from build123d import *

# Parameters (mm, degrees)
REVOLVE_1_ANGLE             = 75
HOLE_WIZARD_M31_D           = 3.4
HOLE_WIZARD_M31_CBORE_D     = 6.05
HOLE_WIZARD_M31_CBORE_DEPTH = 3
FILLET_1_R                  = 2


with BuildPart() as part:
    # Эскиз1 → Повернуть1 (revolve)
    with BuildSketch(Plane.XY):
        Polygon((-52, 0), (-38.5, 0), (-38.5, 5.5), (-48, 5.5), (-48, 10), (-52, 10), align=None)
    revolve(axis=Axis((0, 0, 0), (0, -1, 0)), revolution_arc=REVOLVE_1_ANGLE)

    # Цековка для винта с заклепочной головкой M31 (through all)
    with Locations(Plane(origin=(0, 5.5, 0), x_dir=(1, 0, 0), z_dir=(0, 1, 0))):
        with Locations((-20.75, 35.940054257), (-40.085921791, 10.740990372)):
            CounterBoreHole(HOLE_WIZARD_M31_D / 2, HOLE_WIZARD_M31_CBORE_D / 2, HOLE_WIZARD_M31_CBORE_DEPTH)

    # Скругление1
    fillet_1_edges = [part.edges().sort_by_distance(p)[0] for p in [
        (-9.964533236, 2.75, -37.188144312),
        (-13.458590345, 5, -50.228142967),
        (-52, 5, 0),
        (-38.5, 2.75, 0),
    ]]
    fillet(fillet_1_edges, radius=FILLET_1_R)


solid = part.part
Part model, mm, in its own coordinate system. A direction names the side the tool comes from. Give positions to 0.01 mm unless a question says otherwise; leave off trailing zeros. Order: outer loops, then holes, each group sorted by start corner. A loop starts at its lowest first (then second) coordinate and runs counter-clockwise, first axis right, second up. Notation, with made-up numbers: (-23.5, 73) - (0.5, 73) arc R38 ccw to (0.5, 111) - close; hole circle Ø1 at (58, 83.5). An arc over 180 degrees is marked (long way). Use a Markdown table: item, result.
1) Saw through at B-B on y = 8.5. List the corners of the cut face in (x, z).
Checked values:
| item | result |
|---|---|
| outline | (-51.96, -2.08) arc R52 ccw to (-15.46, -49.65) arc R2 ccw to (-12.93, -48.26) - (-12.42, -46.36) arc R48 cw to (-48, 0) - (-49.96, 0) arc R2 ccw to start |
2) 3-axis set-ups, long thin cutter, end or side, ignore diameter. For faces 4 (the flat face through (-46, 4, 0)), 5 (the flat face through (-39, 2.5, -9)): which of +Z, -Z, +X, -X, +Y, -Y reach the whole face in a straight line?
Checked values:
| item | result |
|---|---|
| face 4 | +Z, +X, -X, +Y, -Y |
| face 5 | +Y |
3) Saw through at A-A on x = -20.75. List the corners of the cut face in (y, z).
Checked values:
| item | result |
|---|---|
| outline | (0, -47.68) - (10, -47.68) - (10, -43.28) - (5.5, -43.28) - (5.5, -38.97) - (2.5, -38.97) - (2.5, -37.64) - (0, -37.64) - close; (0, -34.24) - (2.5, -34.24) - (2.5, -32.92) - (5.5, -32.92) - (5.5, -32.43) - (0, -32.43) - close |
4) Saw through at C-C on z = -17. List the corners of the cut face in (x, y), plus the area to 3 significant figures.
Checked values:
| item | result |
|---|---|
| outline | (-49.14, 0) - (-34.54, 0) - (-34.54, 5.5) - (-44.89, 5.5) - (-44.89, 10) - (-49.14, 10) - close |
| area | 99.4 mm² |
5) Flat gauge pins, fed straight in: P1, Ø5, axis at y = 2.5, z = -19.5, coming from the -X side; P2, Ø3, axis at x = -39.5, z = -11, coming from the +Y side; P3, Ø6.5, axis at x = -20.5, z = -36, coming from the +Y side. Where does each tip first touch, or does it go through?
Checked values:
| item | result |
|---|---|
| P1 | x = -49.14 |
| P2 | y = 2.5 |
| P3 | y = 5.5 |
6) Probe L1, parallel to Y at x = -31.5, z = -24; L2, parallel to Z at x = -23.5, y = 4.5; L3, parallel to Z at x = -20, y = 1.75. List the from-to ranges inside material, lowest first. Write a range as from..to.
Checked values:
| item | result |
|---|---|
| L1 | 0..5.5 |
| L2 | -46.39..-37.2, -34.68..-30.5 |
| L3 | -48..-37.47, -34.41..-32.9 |
7) Two-plate mould, pull along X, no slides. Class faces 1 (the flat face through (-32, 5.5, -23)), 2 (the cylindrical face through (-22.15, 4.02, -38.62)), 3 (the cylindrical face through (-38.347, 7.781, -28.87)): +X half, -X half, draft (parallel to the pull), parting line (faces both ways), or undercut.
Checked values:
| item | result |
|---|---|
| face 1 | draft |
| face 2 | undercut |
| face 3 | +X half |
